Design review of the part built by this model. Coordinates are the model's own, in mm. Face numbers are marked on the shaded views. A direction names the side the tool comes from. Round coordinates to 2 decimals unless told otherwise and drop trailing zeros. Loops run counter-clockwise (first coordinate to the right, second up) from the corner with the lowest first, then second, coordinate; pieces in that order, holes last. Notation, with made-up numbers: (25.5, 75) - (50.5, 75) arc R17 ccw to (50.5, 85) - close; hole circle Ø8 at (27, 65.5). An arc over 180 degrees is marked (long way). Return JSON: item names as keys, results as strings. Group by question number.
(1) The part is to be moulded in two halves that separate along X. For the marked faces 4, 5 and 6, say which applies: pulls with the +X half, pulls with the -X half, needs draft (parallel to the pull), parting line crosses it, or undercut.
(2) Wall thickness on L1, parallel to Y at x = -10, z = 10; L2, parallel to Y at x = -24.3, z = 1.8; L3, parallel to X at y = 1, z = 4.5: over which ranges is each line inside the solid? List them lowest first. Write a range as [from, to].
(3) We need section D-D, the plane y = 24. Write out the cut boundary in (x, z), and give its area (3 significant figures).
(4) We need section C-C, the plane y = 0. Write out the cut boundary in (x, z), and give its area (3 significant figures).
(5) We need section A-A, the plane x = -24.3. Write out the cut boundary in (y, z).
(6) Clearance check with flat-ended pins moving along their axes: pin 1 (2 mm diameter, centred on x = 9.5, z = 1.5, fed in from +Y); pin 2 (11 mm diameter, centred on x = -5, y = 9.5, fed in from +Z); pin 3 (8 mm diameter, centred on x = 0, y = 22, fed in from +Z). State where each tip first meets the part, or that it passes through.
(7) We need section B-B, the plane z = 10.5. Write out the cut boundary in (x, y).
(8) For the marked faces 1, 2 and 3, list the 3-axis set-ups (+Z, -Z, +X, -X, +Y, -Y) from which the entire face can be reached by the end or side of a thin tool; tool diameter is ignored.
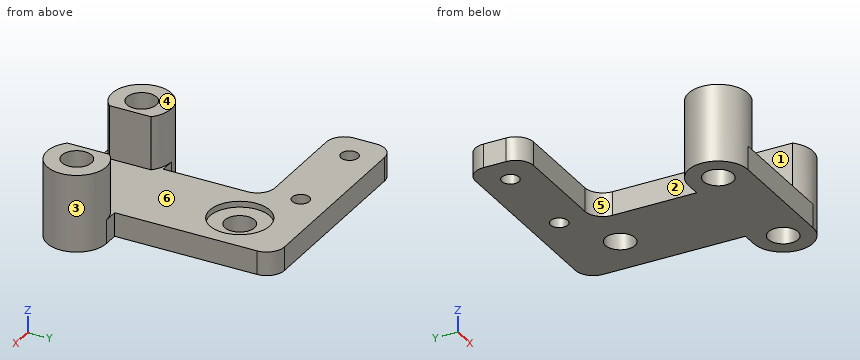
from build123d import *

# Parameters (mm, degrees)
SKETCH_R          = 2.5
SKETCH_R_2        = 1.45
PAD_DEPTH         = 4
SKETCH003_R       = 5
SKETCH003_R_2     = 2.5
PAD001_DEPTH      = 9
SKETCH002_W       = 12.9
SKETCH002_H       = 16.151024
POCKET_DEPTH      = 32.001
POCKET_DEPTH_BACK = 5.001
FILLET_R          = 3
SKETCH004_R       = 5.05
POCKET001_DEPTH   = 1


with BuildPart() as part:
    # Sketch → Pad (new body)
    with BuildSketch(Plane.XY):
        with BuildLine():
            Line((-10, -5), (10, -5))
            ThreePointArc((10, -5), (15, 0), (10, 5))
            Line((7.5, 5), (10, 5))
            Line((7.5, 32), (7.5, 5))
            Line((-7.5, 32), (7.5, 32))
            Line((-29.3, 32), (-7.5, 32))
            Line((-29.3, 22.2), (-29.3, 32))
            Line((-7.5, 22.2), (-29.3, 22.2))
            Line((-7.5, 5), (-7.5, 22.2))
            Line((-7.5, 5), (-10.000009, 5))
            ThreePointArc((-10.000009, 5), (-15, -4e-06), (-10, -5))
        make_face()
        with Locations((-10, 0)):
            Circle(SKETCH_R, mode=Mode.SUBTRACT)
        with Locations((10, 0)):
            Circle(SKETCH_R, mode=Mode.SUBTRACT)
        with Locations((0, 22)):
            Circle(SKETCH_R, mode=Mode.SUBTRACT)
        with Locations((-9.3, 27.2)):
            Circle(SKETCH_R_2, mode=Mode.SUBTRACT)
        with Locations((-24.3, 27.2)):
            Circle(SKETCH_R_2, mode=Mode.SUBTRACT)
    extrude(amount=PAD_DEPTH)

    # Sketch003 (on DatumPlane) → Pad001 (join)
    with BuildSketch(Plane.XY.offset(4)):
        with Locations((-10, 0)):
            Circle(SKETCH003_R)
        with Locations((-10, 0)):
            Circle(SKETCH003_R_2, mode=Mode.SUBTRACT)
        with Locations((10, 0)):
            Circle(SKETCH003_R)
        with Locations((10, 0)):
            Circle(SKETCH003_R_2, mode=Mode.SUBTRACT)
    extrude(amount=PAD001_DEPTH)

    # Sketch002 → Pocket (cut, two sides)
    with BuildSketch(Plane.XZ) as pocket_sk:
        with Locations((0, 12.075512)):
            Rectangle(SKETCH002_W, SKETCH002_H)
    extrude(amount=-POCKET_DEPTH, mode=Mode.SUBTRACT)
    extrude(pocket_sk.sketch, amount=POCKET_DEPTH_BACK, mode=Mode.SUBTRACT)

    # Fillet
    fillet_edges = [part.edges().sort_by_distance(p)[0] for p in [
        (-29.3, 22.2, 2),
        (-29.3, 32, 2),
        (-7.5, 22.2, 2),
        (7.5, 32, 2),
    ]]
    fillet(fillet_edges, radius=FILLET_R)

    # Sketch004 (on Face5 of Fillet) → Pocket001 (cut)
    with BuildSketch(Plane.XY.offset(4)):
        with Locations((0, 22)):
            Circle(SKETCH004_R)
    extrude(amount=-POCKET001_DEPTH, mode=Mode.SUBTRACT)


solid = part.part
Solutions:
{
 "1": {"face 4": "needs draft", "face 5": "pulls with the -X half", "face 6": "undercut"},
 "2": {"L1": "[-5, -2.5], [2.5, 5]", "L2": "[22.2, 25.75], [28.65, 32]", "L3": "[-14.9, -12.29], [-7.71, -6.45], [6.45, 7.71], [12.29, 14.9]"},
 "3": {"outline": "(-29.05, 0) - (-1.5, 0) - (-1.5, 3) - (-4.64, 3) - (-4.64, 4) - (-29.05, 4) - close; (1.5, 0) - (7.5, 0) - (7.5, 4) - (4.64, 4) - (4.64, 3) - (1.5, 3) - close", "area": "128 mm^2"},
 "4": {"outline": "(-15, 0) - (-12.5, 0) - (-12.5, 13) - (-15, 13) - close; (-7.5, 0) - (7.5, 0) - (7.5, 13) - (6.45, 13) - (6.45, 4) - (-6.45, 4) - (-6.45, 13) - (-7.5, 13) - close; (12.5, 0) - (15, 0) - (15, 13) - (12.5, 13) - close", "area": "144 mm^2"},
 "5": {"outline": "(22.2, 0) - (25.75, 0) - (25.75, 4) - (22.2, 4) - close; (28.65, 0) - (32, 0) - (32, 4) - (28.65, 4) - close"},
 "6": {"pin 1": "y = 5", "pin 2": "z = 4", "pin 3": "z = 3"},
 "7": {"outline": "(-6.45, -3.52) - (-6.45, 3.52) arc R5 ccw (long way) to start; (6.45, -3.52) arc R5 ccw (long way) to (6.45, 3.52) - close; hole circle Ø5 at (-10, 0); hole circle Ø5 at (10, 0)"},
 "8": {"face 1": "+Z, +Y, -Y", "face 2": "+Z, -Z, -X", "face 3": "+Z"}
}
